```python
from build123d import *

# Parameters (mm, degrees)
F1_DEPTH = 25
F2_T     = -2.5
F3_W     = 57.5590915978
F3_H     = 17.1818211675
F4_DEPTH = 3
F6_D     = 6.5
F6_DEPTH = 20
F6_TIP   = 1.9527970118
F3_W_2   = 2.5772750378
F3_H_2   = 5.9181824327
F7_DEPTH = 25
F8_R     = 3


with BuildPart() as f1:
    # F0 (on Top) → F1 (new body)
    with BuildSketch(Plane.XY):
        with BuildLine():
            ThreePointArc((-21.8846033079, 32.9097392278), (-21.0659438034, 36.4106418656), (-20.7909114063, 39.9954542518))
            ThreePointArc((-20.7909114063, 39.9954542518), (-21.0659438034, 43.580266638), (-21.8846033079, 47.0811692758))
            ThreePointArc((-21.8846033079, 47.0811692758), (-67.7909114063, 39.9954542518), (-21.8846033079, 32.9097392278))
        make_face()
    extrude(amount=F1_DEPTH)

    # F2
    f2_openings = [f1.faces().sort_by_distance(p)[0] for p in [
        (-44.290911, 39.995454, 25),
    ]]
    offset(amount=F2_T, openings=f2_openings)

    # F3 (on Top) → F4 (join)
    with BuildSketch(Plane.XY):
        with Locations((5.7749990374, 40.5681841075)):
            Rectangle(F3_W, F3_H)
    extrude(amount=F4_DEPTH)

    # F6
    with Locations(Plane(origin=(0, 0, 0), x_dir=(1, 0, 0), z_dir=(0, 0, -1))):
        with Locations((25.1045487821, -41.140910238)):
            Hole(F6_D / 2, depth=F6_DEPTH)
            with Locations((0, 0, -(F6_DEPTH + F6_TIP / 2))):  # 118° drill point
                Cone(0, F6_D / 2, F6_TIP, mode=Mode.SUBTRACT)

    # F3 (on Top) → F7 (cut)
    with BuildSketch(Plane.XY):
        with Locations((-66.2931874394, 39.7090911865)):
            Rectangle(F3_W_2, F3_H_2)
    extrude(amount=F7_DEPTH, mode=Mode.SUBTRACT)

    # F8
    f8_edges = [f1.edges().sort_by_distance(p)[0] for p in [
        (34.554545, 31.977274, 1.5),
        (34.554545, 49.159095, 1.5),
    ]]
    fillet(f8_edges, radius=F8_R)


solid = f1.part
```
Can you work these out from the model? Positions are in its coordinate system, mm. A direction names the side the tool comes from. Give positions to 0.01 mm unless a question says otherwise; leave off trailing zeros. Order: outer loops, then holes, each group sorted by start corner. A loop starts at its lowest first (then second) coordinate and runs counter-clockwise, first axis right, second up. Notation, with made-up numbers: M -35,32.25 L -22,32.25 A12 cw -22,39.25 Z; hole C -13.5,57 d9. An arc over 180 degrees is marked long. Write item = value, one per line. Start each with the question number.
Q1. For faces 1 (the flat face through (-65.005, 40, 1)), 2 (the flat face through (-44, 40, 2.5)), 3 (the flat face through (4, 49.159, 1)), 4 (the flat face through (-66, 36.75, 12)), which set-ups out of +Z, -Z, +X, -X, +Y, -Y let a thin tool reach every point of the face, with its end or its side?
Q2. Suppose I cut it at A-A (z = 4.25). Write out the boundary of the cut face in (x, y), plus the area to 3 significant figures.
Q3. We'd pull the mould along Y, two halves only. Please class faces 5 (the flat face through (-66, 42.668, 12)), 6 (the cylindrical face through (33.7, 32.88, 1.52)), 7 (the cylindrical face through (33.652, 48.304, 1.521)): pulls with the +Y half, pulls with the -Y half, needs draft (parallel to the pull), parting line crosses it, or undercut.
Q4. Suppose I cut it at B-B (x = 27). Write out the boundary of the cut face in (y, z).
Q5. I need wall thicknesses on probe 1 along Z at (x, y) = (-15.5, 45); probe 2 along X at (y, z) = (21.5, 3); probe 3 along X at (y, z) = (23, 20.25). Which ranges of each line are inside material? Lowest first, please. Write a range as [from, to].
Q6. Suppose I cut it at C-C (x = -54). Write out the boundary of the cut face in (y, z), plus the area to 3 significant figures.
Q7. Suppose I cut it at D-D (y = 60). Write out the boundary of the cut face in (x, z), plus the area to 3 significant figures.
Q8. Will these pins go through, and if not, where does the flat tip stop? pin 1 Ø3 at (y, z) = (56.5, 6) entering from -X; pin 2 Ø1.3 at (x, z) = (-66.5, 11.5) entering from +Y; pin 3 Ø1.2 at (y, z) = (40, 1) entering from -X; pin 4 Ø8 at (x, y) = (-26, 22) entering from +Z.
Check result:
q1.face_1 = +Z, -Z
q1.face_2 = +Z
q1.face_3 = +Z, -Z, +X, +Y
q1.face_4 = +Z, -Z, -X
q2.outline = M -67.58,36.87 L -67.58,42.67 L -65.12,42.67 A21 cw long -65.04,36.75 L -67.57,36.75 A23.5 ccw long Z
q2.area = 336 mm2
q3.face_5 = undercut
q3.face_6 = pulls with the -Y half
q3.face_7 = pulls with the +Y half
q4.outline = M 31.98,0 L 38.5,0 L 38.5,3 L 31.98,3 Z; M 43.78,0 L 49.16,0 L 49.16,3 L 43.78,3 Z
q5.probe_1 = [0, 3]
q5.probe_2 = [-58.79, -54.24], [-34.35, -29.79]
q5.probe_3 = [-60.52, -56.63], [-31.96, -28.06]
q6.outline = M 18.59,0 L 61.4,0 L 61.4,25 L 58.62,25 L 58.62,2.5 L 21.37,2.5 L 21.37,25 L 18.59,25 Z
q6.area = 232 mm2
q7.outline = M -56.62,0 L -31.96,0 L -31.96,25 L -37.9,25 L -37.9,2.5 L -50.68,2.5 L -50.68,25 L -56.62,25 Z
q7.area = 329 mm2
q8.pin_1 = -62.38
q8.pin_2 = 49.35
q8.pin_3 = -67.79
q8.pin_4 = 25
